Check sheet for the modelled part. Datum: model origin and axes. Units: mm. Face numbers are marked on the shaded views. A direction names the side the tool comes from. Give positions to 0.01 mm unless a question says otherwise; leave off trailing zeros. Loops run counter-clockwise (first coordinate to the right, second up) from the corner with the lowest first, then second, coordinate; pieces in that order, holes last. Notation, with made-up numbers: M 60,85 L 84,85 A23 ccw 84,111 Z; hole C 0.25,-7 d10. An arc over 180 degrees is marked long. Write each question's results on one line, items separated by ' | '. Start each with the question number.
1. Sectioned sample at B-B on z = 0. Record the cut outline in (x, y), and give its area (3 significant figures).
2. Material ranges on line 1 along Z through (x, y) = (-0.05, 7); line 2 along Y through (x, z) = (1.05, -0.2), recorded low to high.
3. Sectioned sample at A-A on x = 0. Record the cut outline in (y, z).
4. Sectioned sample at D-D on y = 10.5. Record the cut outline in (x, z), and give its area (3 significant figures).
5. Go/stop test with flat-tipped pins: pin 1 (1.5 mm diameter, centred on x = 0, y = 4, fed in from +Z); pin 2 (1 mm diameter, centred on y = 6.5, z = 0, fed in from +X). Record where each tip stops, or that it passes through.
6. Sectioned sample at C-C on y = 6. Record the cut outline in (x, z), and give its area (3 significant figures).
7. Tool access check on the marked faces 1 and 2. Record the directions out of +Z, -Z, +X, -X, +Y, -Y that give a thin tool (end or side, any length) a straight path to the whole face; none if there is none.
```python
from build123d import *


with BuildPart() as part:
    # Esquisse1 → Révolution1 (revolve)
    with BuildSketch(Plane.XY, mode=Mode.PRIVATE) as r_volution1_sk:
        with BuildLine():
            Line((0, 0), (1.5, 0))
            Line((1.5, 0), (1.5, 3))
            Line((1.5, 3), (1, 3))
            Line((1, 3), (1, 10.25))
            Line((1, 10.25), (0.75, 10.25))
            Line((0.75, 10.25), (0.75, 10.75))
            Line((0.75, 10.75), (1, 10.75))
            Line((1, 10.75), (1, 11.25))
            ThreePointArc((1, 11.25), (0.926776695, 11.426776695), (0.75, 11.5))
            Line((0.75, 11.5), (0, 11.5))
            Line((0, 11.5), (0, 0))
        make_face()
    revolve(r_volution1_sk.sketch.rotate(Axis((0, 0, 0), (0, 1, 0)), 90), axis=Axis((0, 0, 0), (0, 1, 0)))


solid = part.part
```
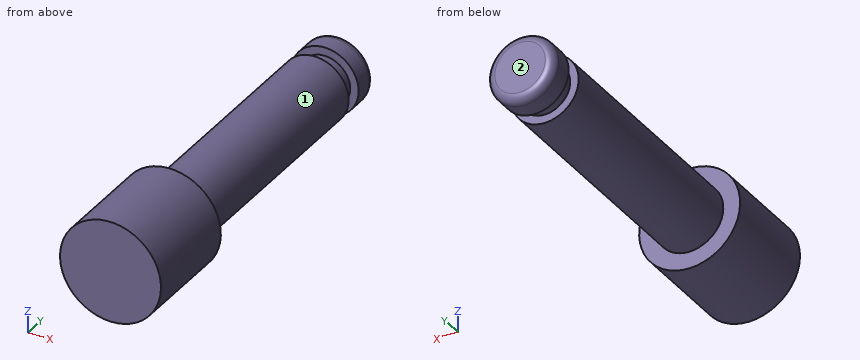
Output values:
1) outline: M -1.5,0 L 1.5,0 L 1.5,3 L 1,3 L 1,10.25 L 0.75,10.25 L 0.75,10.75 L 1,10.75 L 1,11.25 A0.25 ccw 0.75,11.5 L -0.75,11.5 A0.25 ccw -1,11.25 L -1,10.75 L -0.75,10.75 L -0.75,10.25 L -1,10.25 L -1,3 L -1.5,3 Z | area: 25.7 mm2
2) line 1: -1 to 1 | line 2: 0 to 3
3) outline: M 0,-1.5 L 3,-1.5 L 3,-1 L 10.25,-1 L 10.25,-0.75 L 10.75,-0.75 L 10.75,-1 L 11.25,-1 A0.25 ccw 11.5,-0.75 L 11.5,0.75 A0.25 ccw 11.25,1 L 10.75,1 L 10.75,0.75 L 10.25,0.75 L 10.25,1 L 3,1 L 3,1.5 L 0,1.5 Z
4) outline: C 0,0 d1.5 | area: 1.77 mm2
5) pin 1: z = 1 | pin 2: x = 1
6) outline: C 0,0 d2 | area: 3.14 mm2
7) face 1: +Y | face 2: +Z, -Z, +X, -X, +Y
